Part model, mm, in its own coordinate system. A direction names the side the tool comes from. Give positions to 0.01 mm unless a question says otherwise; leave off trailing zeros. Order: outer loops, then holes, each group sorted by start corner. A loop starts at its lowest first (then second) coordinate and runs counter-clockwise, first axis right, second up. Notation, with made-up numbers: M 89,24 L 136,24 A27 ccw 136,54 Z; hole C -36.75,50.5 d8. An arc over 180 degrees is marked long. Answer as a JSON object with one key per item and string values.
from build123d import *

# Parameters (mm, degrees)
REVOLVE1_ANGLE      = 180
SKETCH8_R           = 7.5
BOSS_EXTRUDE1_DEPTH = 5
BOSS_EXTRUDE1_TAPER = 30
FILLET3_R           = 5
SHELL7_T            = -0.5
CUT_EXTRUDE1_DEPTH  = 23
CUT_EXTRUDE4_DEPTH  = 2.5


with BuildPart() as part:
    # Sketch5 → Revolve1 (revolve)
    with BuildSketch(Plane(origin=(0, 0, 0), x_dir=(1, 0, 0), z_dir=(0, 1, 0))):
        with BuildLine():
            Line((-15, 0), (0, 0))
            ThreePointArc((0, 0), (-7.5, -7.5), (-15, 0))
        make_face()
    revolve(axis=Axis((0, 0, 0), (-1, 0, 0)), revolution_arc=REVOLVE1_ANGLE)

    # Sketch8 → Boss-Extrude1 (add)
    with BuildSketch(Plane.XZ):
        with Locations((-7.5, 0)):
            Circle(SKETCH8_R)
    extrude(amount=BOSS_EXTRUDE1_DEPTH, taper=BOSS_EXTRUDE1_TAPER)

    # Fillet3
    fillet3_edges = [part.edges().sort_by_distance(p)[0] for p in [
        (-7.5, 0, -7.5),
    ]]
    fillet(fillet3_edges, radius=FILLET3_R)

    # Shell7
    shell7_openings = [part.faces().sort_by_distance(p)[0] for p in [
        (-7.5, -5, 0),
    ]]
    offset(amount=SHELL7_T, openings=shell7_openings, kind=Kind.INTERSECTION)

    # Sketch9 → Cut-Extrude1 (cut)
    with BuildSketch(Plane(origin=(0, 0, 0), x_dir=(0, 0, -1), z_dir=(1, 0, 0))):
        with BuildLine():
            Line((1.557300456, -3.245702646), (2.220059838, 1.52969178))
            Line((2.220059838, 1.52969178), (-2.220059838, 1.52969178))
            Line((-2.220059838, 1.52969178), (-1.556069246, -2.994983603))
            ThreePointArc((-1.556069246, -2.994983603), (-0.125361033, -4.684691185), (1.557300456, -3.245702646))
        make_face()
    extrude(amount=-CUT_EXTRUDE1_DEPTH, mode=Mode.SUBTRACT)

    # Sketch11 → Cut-Extrude4 (cut)
    with BuildSketch(Plane(origin=(0, 7.5, 0), x_dir=(1, 0, 0), z_dir=(0, 1, 0))):
        Polygon((-7.5, 6.89001607), (-0.60998393, 6.89001607), (-0.60998393, -6.89001607), (-14.767195706, -6.89001607), (-14.767195706, 0), (-14.767195706, 6.89001607), align=None)
    extrude(amount=-CUT_EXTRUDE4_DEPTH, mode=Mode.SUBTRACT)


solid = part.part
1. Cut at A-A on y = -3.75. Give the cut face in (x, z).
Worked answers:
{"outline": "M -12.64,-1.43 A5.33 ccw -2.36,-1.43 L -2.96,-1.43 A4.76 cw -12.04,-1.43 Z; M -12.64,1.43 L -12.04,1.43 A4.76 cw -2.96,1.43 L -2.36,1.43 A5.33 ccw Z"}
2. Two-plate mould, pull along X, no slides. Class faces 1 (the conical face through (-3.68, -4.82, -1.59)), 2 (the conical face through (-3.01, -4.83, 1.42)), 3 (the flat face through (-1.193, -0.869, -1.887)): +X half, -X half, draft (parallel to the pull), parting line (faces both ways), or undercut.
Worked answers:
{"face 1": "undercut", "face 2": "parting line", "face 3": "draft"}
3. Pin check, flat tips, straight feed: P1, Ø4, axis at x = -12.5, y = 2, coming from the -Z side; P2, Ø1, axis at x = -14, z = 0, coming from the -Y side; P3, Ø1, axis at x = -5, z = 3.5, coming from the +Y side. Stop position of each tip, or through.
Worked answers:
{"P1": "stops at z = -6.59", "P2": "stops at y = 1.53", "P3": "stops at y = -3.67"}
4. Cut at B-B on z = 0. State how many separate pieces and enclosed holes the cut face has, plus the area to 3 significant figures.
Worked answers:
{"separate pieces": "4", "enclosed holes": "0", "area": "4.32 mm^2"}
5. Probe line 1 along X through (y, z) = (3.75, 2.75); line 2 along Z through (x, y) = (-13.5, 0.25); line 3 along Z through (x, y) = (-9.75, 0.5). List the from-to ranges inside material, lowest first.
Worked answers:
{"line 1": "x = -13.38 to -12.73, -2.27 to -1.62", "line 2": "z = -4.06 to -3.06, 3.06 to 4.06", "line 3": "z = -6.92 to -6.39, 6.39 to 6.92"}
6. Which spindle directions (+Z, -Z, +X, -X, +Y, -Y) get a long thin tool onto all of the face, cutting with end or side? Do faces 4 (the cylindrical face through (-2.9, -4.68, 0.16)), 5 (the flat face through (-11, 5, 4)). Say none if no direction does.
Worked answers:
{"face 4": "+X, -X", "face 5": "+Z, -Z, +X, -X, +Y"}
